Geometry: final body of the model. Coordinates: model frame, mm. Face numbers are marked on the shaded views. Round coordinates to 2 decimals unless told otherwise and drop trailing zeros. One line per item, written item: value. Start each with the question number.
from build123d import *

# Parameters (mm, degrees)
ESQUISSE1_W             = 96
ESQUISSE1_H             = 86
BOSS_EXTRU_1_DEPTH      = 5
BOSS_EXTRU_4_DEPTH      = 30
CONG_2_R                = 5
ESQUISSE4_R             = 1.6
ENL_V_MAT_EXTRU_1_DEPTH = 10
BOSS_EXTRU_17_DEPTH     = 30
ESQUISSE22_R            = 1.5
ENL_V_MAT_EXTRU_5_DEPTH = 10
BOSS_EXTRU_14_DEPTH     = 20
BOSS_EXTRU_15_DEPTH     = 30
ESQUISSE17_R            = 1.5
ENL_V_MAT_EXTRU_3_DEPTH = 10
BOSS_EXTRU_16_DEPTH     = 30
ESQUISSE19_R            = 1.5
ENL_V_MAT_EXTRU_4_DEPTH = 10
CONG_6_R                = 5
CONG_14_R               = 3
TROUM3_D                = 3.4


# Some blends are built 0.0001 mm under size
with BuildPart() as part:
    # Esquisse1 → Boss.-Extru.1 (new body)
    with BuildSketch(Plane.XY):
        with Locations((2.2, -13.159463773)):
            Rectangle(ESQUISSE1_W, ESQUISSE1_H)
    extrude(amount=BOSS_EXTRU_1_DEPTH)

    # Esquisse2 → Boss.-Extru.4 (add)
    with BuildSketch(Plane.XY.offset(5)):
        Polygon((-45.8, 29.840536227), (-45.8, 14.840536227), (-44.8, 14.840536227), (-44.8, 19.840536227), (-41.3, 19.840536227), (-41.3, 14.840536227), (-40.3, 14.840536227), (-40.3, 24.340536227), (-30.8, 24.340536227), (-30.8, 25.340536227), (-35.8, 25.340536227), (-35.8, 28.840536227), (-30.8, 28.840536227), (-30.8, 29.840536227), align=None)
    extrude(amount=BOSS_EXTRU_4_DEPTH)

    # Congé2
    cong_2_edges = [part.edges().sort_by_distance(p)[0] for p in [
        (-45.8, -13.159463773, 0),
        (2.2, -56.159463773, 0),
        (50.2, -13.159463773, 0),
        (2.2, 29.840536227, 0),
    ]]
    fillet(cong_2_edges, radius=CONG_2_R - 0.0001)  # a hair under: the kernel refuses the full size

    # Esquisse4 → Enlèv. mat.-Extru.1 (cut)
    with BuildSketch(Plane.XY.offset(35)):
        with Locations((-42.3, 26.340536227)):
            Circle(ESQUISSE4_R)
    extrude(amount=-ENL_V_MAT_EXTRU_1_DEPTH, mode=Mode.SUBTRACT)

    # Esquisse21 → Boss.-Extru.17 (add)
    with BuildSketch(Plane.XY.offset(5)):
        Polygon((-45.8, -56.159463773), (-45.8, -41.159463773), (-44.8, -41.159463773), (-44.8, -46.159463773), (-41.3, -46.159463773), (-41.3, -41.159463773), (-40.3, -41.159463773), (-40.3, -50.659463773), (-30.8, -50.659463773), (-30.8, -51.659463773), (-35.8, -51.659463773), (-35.8, -55.159463773), (-30.8, -55.159463773), (-30.8, -56.159463773), align=None)
    extrude(amount=BOSS_EXTRU_17_DEPTH)

    # Esquisse22 → Enlèv. mat.-Extru.5 (cut)
    with BuildSketch(Plane.XY.offset(35)):
        with Locations((-42.3, -52.659463773)):
            Circle(ESQUISSE22_R)
    extrude(amount=-ENL_V_MAT_EXTRU_5_DEPTH, mode=Mode.SUBTRACT)

    # Esquisse14 → Boss.-Extru.14 (add)
    with BuildSketch(Plane.XY.offset(5)):
        Polygon((-45.8, -56.159463773), (-45.8, -41.159463773), (-44.8, -41.159463773), (-44.8, -46.159463773), (-41.3, -46.159463773), (-41.3, -41.159463773), (-40.3, -41.159463773), (-40.3, -50.659463773), (-30.8, -50.659463773), (-30.8, -51.659463773), (-35.8, -51.659463773), (-35.8, -55.159463773), (-30.8, -55.159463773), (-30.8, -56.159463773), align=None)
    extrude(amount=BOSS_EXTRU_14_DEPTH)

    # Esquisse16 → Boss.-Extru.15 (add)
    with BuildSketch(Plane.XY.offset(5)):
        Polygon((50.2, 29.840536227), (35.2, 29.840536227), (35.2, 28.840536227), (40.2, 28.840536227), (40.2, 25.340536227), (35.2, 25.340536227), (35.2, 24.340536227), (44.7, 24.340536227), (44.7, 14.840536227), (45.7, 14.840536227), (45.7, 19.840536227), (49.2, 19.840536227), (49.2, 14.840536227), (50.2, 14.840536227), align=None)
    extrude(amount=BOSS_EXTRU_15_DEPTH)

    # Esquisse17 → Enlèv. mat.-Extru.3 (cut)
    with BuildSketch(Plane.XY.offset(35)):
        with Locations((46.7, 26.340536227)):
            Circle(ESQUISSE17_R)
    extrude(amount=-ENL_V_MAT_EXTRU_3_DEPTH, mode=Mode.SUBTRACT)

    # Esquisse18 → Boss.-Extru.16 (add)
    with BuildSketch(Plane.XY.offset(5)):
        Polygon((50.2, -56.159463773), (50.2, -41.159463773), (49.2, -41.159463773), (49.2, -46.159463773), (45.7, -46.159463773), (45.7, -41.159463773), (44.7, -41.159463773), (44.7, -50.659463773), (35.2, -50.659463773), (35.2, -51.659463773), (40.2, -51.659463773), (40.2, -55.159463773), (35.2, -55.159463773), (35.2, -56.159463773), align=None)
    extrude(amount=BOSS_EXTRU_16_DEPTH)

    # Esquisse19 → Enlèv. mat.-Extru.4 (cut)
    with BuildSketch(Plane.XY.offset(35)):
        with Locations((46.7, -52.659463773)):
            Circle(ESQUISSE19_R)
    extrude(amount=-ENL_V_MAT_EXTRU_4_DEPTH, mode=Mode.SUBTRACT)

    # Congé6
    # the kernel refuses this fillet: 5 mm, written as the material it takes off along each edge
    with BuildSketch(Plane(origin=(-40.8, 24.840536227, 0), x_dir=(-1, 0, 0), z_dir=(0, -1, 0))) as cong_6_piece_1:
        with BuildLine():
            CenterArc((0.0001, -4.9999), 4.9999, 0, 90)
            Line((5, -4.9999), (5, 0))
            Line((5, 0), (0.0001, 0))
        make_face()
    revolve(axis=Axis((-40.8, 24.840536227, 0), (0, 0, -1)), revolution_arc=90, mode=Mode.SUBTRACT)
    with BuildSketch(Plane(origin=(45.2, 24.840536227, 0), x_dir=(0, 1, 0), z_dir=(-1, 0, 0))) as cong_6_piece_2:
        with BuildLine():
            CenterArc((0.0001, -4.9999), 4.9999, 0, 90)
            Line((5, -4.9999), (5, 0))
            Line((5, 0), (0.0001, 0))
        make_face()
    revolve(axis=Axis((45.2, 24.840536227, 0), (0, 0, -1)), revolution_arc=90, mode=Mode.SUBTRACT)
    with BuildSketch(Plane(origin=(-40.8, -51.159463773, 0), x_dir=(0, -1, 0), z_dir=(1, 0, 0))) as cong_6_piece_3:
        with BuildLine():
            CenterArc((0.0001, -4.9999), 4.9999, 0, 90)
            Line((5, -4.9999), (5, 0))
            Line((5, 0), (0.0001, 0))
        make_face()
    revolve(axis=Axis((-40.8, -51.159463773, 0), (0, 0, -1)), revolution_arc=90, mode=Mode.SUBTRACT)
    with BuildSketch(Plane(origin=(45.2, -51.159463773, 0), x_dir=(1, 0, 0), z_dir=(0, 1, 0))) as cong_6_piece_4:
        with BuildLine():
            CenterArc((0.0001, -4.9999), 4.9999, 0, 90)
            Line((5, -4.9999), (5, 0))
            Line((5, 0), (0.0001, 0))
        make_face()
    revolve(axis=Axis((45.2, -51.159463773, 0), (0, 0, -1)), revolution_arc=90, mode=Mode.SUBTRACT)
    with BuildSketch(Plane(origin=(50.2, 29.840536227, 0), x_dir=(0, -1, 0), z_dir=(0, 0, 1)), Plane(origin=(50.2, -56.159463773, 0), x_dir=(-1, 0, 0), z_dir=(0, 0, 1)), Plane(origin=(-45.8, -56.159463773, 47.5), x_dir=(1, 0, 0), z_dir=(0, 0, -1)), Plane(origin=(-45.8, 29.840536227, 47.5), x_dir=(0, -1, 0), z_dir=(0, 0, -1))) as cong_6_piece_5:
        with BuildLine():
            CenterArc((CONG_6_R, -CONG_6_R), CONG_6_R, 90, 90)
            Line((0, -CONG_6_R), (0, 0))
            Line((0, 0), (CONG_6_R, 0))
        make_face()
    extrude(amount=47.5, mode=Mode.SUBTRACT)

    # Congé14
    cong_14_edges = [part.edges().sort_by_distance(p)[0] for p in [
        (39.95, 24.340536227, 5),
        (44.7, 19.590536227, 5),
        (44.7, 24.340536227, 20),
        (-40.3, 19.590536227, 5),
        (44.7, -45.909463773, 5),
        (-35.55, 24.340536227, 5),
        (39.95, -50.659463773, 5),
        (44.7, -50.659463773, 20),
        (-40.3, 24.340536227, 20),
        (-35.55, -50.659463773, 5),
        (-40.3, -45.909463773, 5),
        (-40.3, -50.659463773, 20),
    ]]
    fillet(cong_14_edges, radius=CONG_14_R)

    # TrouM3 (through all)
    with Locations(Plane.XY.offset(5)):
        with Locations((-9.71, 10.960536227), (41.09, -4.279463773), (-10.98, -37.299463773), (-4.517514421, -19.876978194), (-4.517514421, -6.441949352), (8.917514421, -6.441949352), (8.917514421, -19.876978194)):
            Hole(TROUM3_D / 2)


solid = part.part
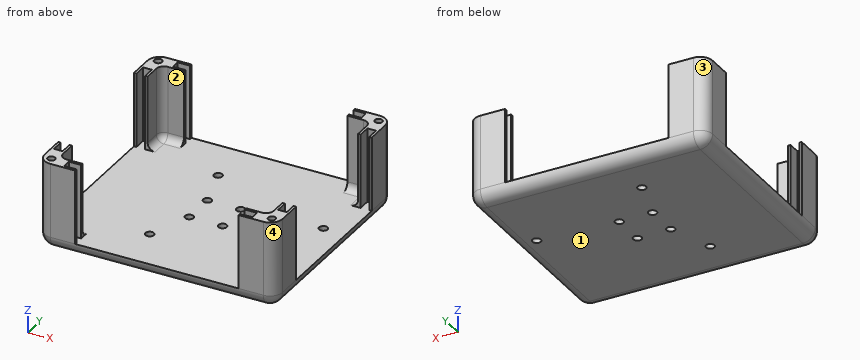
(1) Pull-direction query (Y, two-part tool) for the marked faces 1, 2, 3 and 4; classes: pulls with the +Y half, pulls with the -Y half, needs draft (parallel to the pull), parting line crosses it, or undercut.
(2) Line query: probe 1 along X at (y, z) = (21, 23.5); probe 2 along Y at (x, z) = (-42.3, 30); probe 3 along X at (y, z) = (-51.5, 12.5). Output: solid intervals per line, ascending.
(3) Pin query (flat end, axial travel): pin 1 (0.5 mm diameter, centred on x = -45.5, z = 21.5, fed in from -Y); pin 2 (10 mm diameter, centred on y = 7, z = 30, fed in from -X); pin 3 (4 mm diameter, centred on x = -1, y = -23, fed in from -Z); pin 4 (3 mm diameter, centred on x = 47, z = 17, fed in from +Y). Return the tip coordinate at first contact, or that it passes through.
(4) Section query B-B (z = 29). Count the separate pieces of the cut face and the enclosed holes in it, and give its area (3 significant figures).
Results list:
1. face 1: needs draft
1. face 2: undercut
1. face 3: pulls with the +Y half
1. face 4: pulls with the -Y half
2. probe 1: x = -45.8 to -40.3, 44.7 to 50.2
2. probe 2: y = -55.93 to -54.16, -51.16 to -46.16, 19.84 to 24.74, 27.94 to 29.61
2. probe 3: x = -45.79 to -30.8, 35.2 to 50.19
3. pin 1: stops at y = -53.44
3. pin 2: passes through
3. pin 3: stops at z = 0
3. pin 4: stops at y = 29.83
4. separate pieces: 4
4. enclosed holes: 4
4. area: 356 mm^2
